```python
from build123d import *

# Parameters (mm, degrees)
SKETCH1_R           = 12.5
BOSS_EXTRUDE1_DEPTH = 3
SKETCH3_R           = 1
BOSS_EXTRUDE2_DEPTH = 3
SKETCH4_R           = 7
BOSS_EXTRUDE3_DEPTH = 13
CUT_EXTRUDE1_REACH  = 23.943
SKETCH5_R           = 6
FILLET2_R           = 0.5
FILLET3_R           = 0.5


with BuildPart() as part:
    # Sketch1 → Boss-Extrude1 (new body)
    with BuildSketch(Plane(origin=(0, 0, 0), x_dir=(1, 0, 0), z_dir=(0, 1, 0))):
        with Locations(Location((0, 0, 0), (0, 0, 270))):
            Circle(SKETCH1_R)
        with BuildLine():
            Line((1.5, 2), (4.5, 2))
            ThreePointArc((4.5, 2), (4.853553391, 1.853553391), (5, 1.5))
            Line((5, 1.5), (5, -1.5))
            ThreePointArc((5, -1.5), (4.853553391, -1.853553391), (4.5, -2))
            Line((4.5, -2), (1.5, -2))
            ThreePointArc((1.5, -2), (0, -2.5), (-1.5, -2))
            Line((-1.5, -2), (-4.5, -2))
            ThreePointArc((-4.5, -2), (-4.853553391, -1.853553391), (-5, -1.5))
            Line((-5, -1.5), (-5, 1.5))
            ThreePointArc((-5, 1.5), (-4.853553391, 1.853553391), (-4.5, 2))
            Line((-4.5, 2), (-1.5, 2))
            ThreePointArc((-1.5, 2), (0, 2.5), (1.5, 2))
        make_face(mode=Mode.SUBTRACT)
    extrude(amount=BOSS_EXTRUDE1_DEPTH)

    # Sketch3 → Boss-Extrude2 (add)
    with BuildSketch(Plane.XZ):
        with Locations(Location((-10.5, 0, 0), (0, 0, 90))):
            Circle(SKETCH3_R)
    extrude(amount=BOSS_EXTRUDE2_DEPTH)

    # Sketch4 → Boss-Extrude3 (add)
    with BuildSketch(Plane.XZ):
        with Locations(Location((0, 0, 0), (0, 0, 90))):
            Circle(SKETCH4_R)
    extrude(amount=BOSS_EXTRUDE3_DEPTH)

    # Sketch5 → Cut-Extrude1 (cut, up to next)
    with BuildSketch(Plane(origin=(0, 0, 0), x_dir=(1, 0, 0), z_dir=(0, 1, 0)), mode=Mode.PRIVATE) as cut_extrude1_sk1:
        with Locations(Location((0, 0, 0), (0, 0, 270))):
            Circle(SKETCH5_R)
    cut_extrude1_tool1 = extrude(cut_extrude1_sk1.sketch, amount=-CUT_EXTRUDE1_REACH, mode=Mode.PRIVATE) & part.part
    add(cut_extrude1_tool1.solids().sort_by_distance((0, 0, 0))[0], mode=Mode.SUBTRACT)

    # Fillet2
    fillet2_edges = [part.edges().sort_by_distance(p)[0] for p in [
        (0, 0, -12.5),
        (0, 3, -12.5),
    ]]
    fillet(fillet2_edges, radius=FILLET2_R)

    # Fillet3
    fillet3_edges = [part.edges().sort_by_distance(p)[0] for p in [
        (0, -13, -7),
    ]]
    fillet(fillet3_edges, radius=FILLET3_R)


solid = part.part
```
Geometry check sheet. Reference: the model listing, model coordinates, mm. A direction names the side the tool comes from. Give positions to 0.01 mm unless a question says otherwise; leave off trailing zeros. Order: outer loops, then holes, each group sorted by start corner. A loop starts at its lowest first (then second) coordinate and runs counter-clockwise, first axis right, second up. Notation, with made-up numbers: (33.5, -28.5) - (92.5, -28.5) arc R11 cw to (92.5, -11.5) - close; hole circle Ø3 at (26, -19). An arc over 180 degrees is marked (long way). Write item = value, one per line. Start each with the question number.
1) Scan lines: L1, parallel to X at y = -6, z = 0; L2, parallel to Y at x = 10.75, z = -3.5; L3, parallel to X at y = -7.5, z = -1.25. Record each from-to range of solid material in increasing order.
2) Section check C-C (y = -4). Enter the section's corners in (x, z).
3) Section check B-B (z = 0). Enter the section's corners in (x, y).
4) Draft check along Z on faces 1 (the flat face through (-3, 1, 2)), 2 (the cylindrical face through (3.755, 1.486, 11.923)), 3 (the flat face through (3, 1, 2)), 4 (the flat face through (6, -13, 2)). Enter one of: released by +Z, released by -Z, zero draft, split by the parting line, or undercut.
5) Section check A-A (x = 0). Enter the section's corners in (y, z), then the cut area to 3 significant figures.
6) Access from +Z, -Z, +X, -X, +Y, -Y to the whole of each face (thin tool, end or side, straight path). Record for faces 5 (the cylindrical face through (6.834, -6.162, -1.517)), 6 (the flat face through (3, 1, -2)), 7 (the flat face through (0, 3, -3)), 8 (the flat face through (-11, -3, 0)).
7) Gauge pin test, flat ends, axial feed: pin 1 Ø2.5 at (x, y) = (-3, 2) entering from +Z; pin 2 Ø3 at (y, z) = (-3, 5) entering from -X; pin 3 Ø1.5 at (x, z) = (-7, 8.5) entering from -Y. Record the tip position at first contact, or that the pin passes through.
Geometry check:
q1.L1 = -7 to -6, 6 to 7
q1.L2 = 0 to 3
q1.L3 = -6.89 to -5.87, 5.87 to 6.89
q2.outline = circle Ø14 at (0, 0); hole circle Ø12 at (0, 0)
q3.outline = (-12.5, 0.5) arc R0.5 ccw to (-12, 0) - (-11.5, 0) - (-11.5, -3) - (-9.5, -3) - (-9.5, 0) - (-7, 0) - (-7, -12.5) arc R0.5 ccw to (-6.5, -13) - (-6, -13) - (-6, 0) - (-5, 0) - (-5, 3) - (-12, 3) arc R0.5 ccw to (-12.5, 2.5) - close; (5, 0) - (6, 0) - (6, -13) - (6.5, -13) arc R0.5 ccw to (7, -12.5) - (7, 0) - (12, 0) arc R0.5 ccw to (12.5, 0.5) - (12.5, 2.5) arc R0.5 ccw to (12, 3) - (5, 3) - close
q4.face_1 = undercut
q4.face_2 = split by the parting line
q4.face_3 = undercut
q4.face_4 = zero draft
q5.outline = (-13, -6.5) arc R0.5 ccw to (-12.5, -7) - (0, -7) - (0, -12) arc R0.5 ccw to (0.5, -12.5) - (2.5, -12.5) arc R0.5 ccw to (3, -12) - (3, -2.5) - (0, -2.5) - (0, -6) - (-13, -6) - close; (-13, 6) - (0, 6) - (0, 2.5) - (3, 2.5) - (3, 12) arc R0.5 ccw to (2.5, 12.5) - (0.5, 12.5) arc R0.5 ccw to (0, 12) - (0, 7) - (-12.5, 7) arc R0.5 ccw to (-13, 6.5) - close
q5.area = 85.7 mm2
q6.face_5 = -Y
q6.face_6 = +Y, -Y
q6.face_7 = +Z, -Z, +X, -X, +Y
q6.face_8 = +Z, -Z, -X, -Y
q7.pin_1 = 12.38
q7.pin_2 = -6.06
q7.pin_3 = 0
